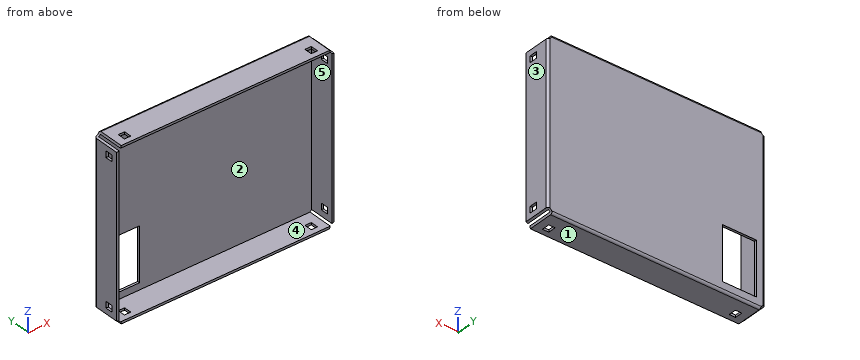
Autodesk Inventor part; units mm, degrees
ref_plane "YZ Plane" through (0, 0, 0) normal (1, 0, 0) x (0, 1, 0)
ref_plane "XZ Plane" through (0, 0, 0) normal (0, 1, 0) x (-1, 0, 0)
ref_plane "XY Plane" through (0, 0, 0) normal (0, 0, 1) x (1, 0, 0)
sketch "Sketch3" plane through (0, 0, 0) normal (0, 1, 0) x (-1, 0, 0)
  line L0 (23, 18.5) -> (-23, 18.5)
  line L1 (-24, 17.5) -> (-24, -17.5)
  line L2 (-23, -18.5) -> (23, -18.5)
  line L3 (24, -17.5) -> (24, 17.5)
  line L4 (24, 18.5) -> (-24, -18.5) construction
  circle A0 centre (24, 18.5) radius 1
  circle A1 centre (24, -18.5) radius 1
  circle A2 centre (-24, -18.5) radius 1
  circle A3 centre (-24, 18.5) radius 1
  point P0 (0, 0)
  dimension "d21" = 2
  dimension "d22" = 2
  dimension "d23" = 2
  dimension "d24" = 2
extrude "Extrusion3" add sketch "Sketch3" along normal blind 0.5 contours A0 L3 A1 L2 A2 L1 A3 L0
sketch "Sketch6" plane through (0, 0, 0) normal (0, -1, 0) x (1, 0, 0)
  line L0 (-23, 18.5) -> (23, 18.5)
  line L1 (-23, 18.5) -> (23, 18.5)
  line L2 (24, 17.5) -> (24, -17.5)
  line L3 (24, 17.5) -> (24, -17.5)
  line L4 (-24, -17.5) -> (-24, 17.5)
  line L5 (-24, -17.5) -> (-24, 17.5)
  circle A0 centre (-24, 18.5) radius 1
  circle A1 centre (24, 18.5) radius 1
  circle A2 centre (24, -18.5) radius 1
  circle A3 centre (-24, -18.5) radius 1
  line L6 (23.5, -17.634) -> (23.5, 17.634)
  line L7 (-23.134, 18) -> (23.134, 18)
  line L8 (-23.5, -17.634) -> (-23.5, 17.634)
  line L9 (23, -18.5) -> (-23, -18.5)
  line L10 (-23, -18.5) -> (23, -18.5)
  line L11 (23.134, -18) -> (-23.134, -18)
  point P0 (0, 0)
  dimension "d45" = 0.5
  dimension "d46" = 0.5
  dimension "d48" = 2
  dimension "d49" = 0.5
extrude "Extrusion5" add sketch "Sketch6" along normal blind 5.5 contours L0 A1 L7 A0 | A0 L8 A3 L4 | L2 A2 L6 A1 | A3 L11 A2 L9
sketch "Sketch7" plane through (-23, 0.5, 18.5) normal (0, 0, 1) x (1, 0, 0)
  line L0 (42.9, -3.1) -> (44.3, -3.1)
  line L1 (44.3, -3.1) -> (44.3, -4.8)
  line L2 (44.3, -4.8) -> (42.9, -4.8)
  line L3 (42.9, -4.8) -> (42.9, -3.1)
  line L4 (0, 0) -> (46, 0)
  line L5 (46, -6) -> (46, 0)
  line L6 (1.7, -3.1) -> (3.1, -3.1)
  line L7 (3.1, -3.1) -> (3.1, -4.8)
  line L8 (3.1, -4.8) -> (1.7, -4.8)
  line L9 (1.7, -4.8) -> (1.7, -3.1)
  line L10 (0, 0) -> (0, -6)
  point P0 (23, -0.5)
  dimension "d52" = 1.4
  dimension "d53" = 1.7
  dimension "d54" = 3.1
  dimension "d55" = 1.7
  dimension "d56" = 1.4
  dimension "d57" = 1.7
  dimension "d58" = 3.1
  dimension "d59" = 1.7
extrude "Extrusion6" cut sketch "Sketch7" against normal up to surface (37 mm away)
sketch "Sketch8" plane through (24, 0.5, 17.5) normal (1, 0, 0) x (0, 0, -1)
  line L0 (32.4, -3.1) -> (33.8, -3.1)
  line L1 (33.8, -3.1) -> (33.8, -4.8)
  line L2 (33.8, -4.8) -> (32.4, -4.8)
  line L3 (32.4, -4.8) -> (32.4, -3.1)
  line L4 (0, 0) -> (35, 0)
  line L5 (35, -6) -> (35, 0)
  line L6 (1.2, -3.1) -> (2.6, -3.1)
  line L7 (2.6, -3.1) -> (2.6, -4.8)
  line L8 (2.6, -4.8) -> (1.2, -4.8)
  line L9 (1.2, -4.8) -> (1.2, -3.1)
  line L10 (0, -6) -> (0, 0)
  point P0 (17.5, -0.5)
  dimension "d62" = 1.4
  dimension "d63" = 1.7
  dimension "d64" = 3.1
  dimension "d65" = 1.2
  dimension "d66" = 1.4
  dimension "d67" = 1.7
  dimension "d68" = 3.1
  dimension "d69" = 1.2
extrude "Extrusion7" cut sketch "Sketch8" against normal up to surface (48 mm away)
sketch "Sketch9" plane through (0, 0.5, 0) normal (0, 1, 0) x (1, 0, 0)
  line L0 (-22, 4.7) -> (-14.5, 4.7)
  line L1 (-14.5, 4.7) -> (-14.5, 16.5)
  line L2 (-14.5, 16.5) -> (-22, 16.5)
  line L3 (-22, 16.5) -> (-22, 4.7)
  line L4 (-24, 17.5) -> (-24, -17.5)
  line L5 (23, 18.5) -> (-23, 18.5)
  point P0 (0, 0)
  dimension "d74" = 7.5
  dimension "d75" = 11.8
  dimension "d76" = 2
  dimension "d77" = 2
extrude "Extrusion8" cut sketch "Sketch9" against normal up to surface (0.5 mm away)
fillet "Fillet1" radius 0.5 4 edges at (0, 0.5, -18.5) (24, 0.5, 0) (0, 0.5, 18.5) (-24, 0.5, 0)
properties part number "metal_cover_connector"
The listing builds one solid part. Answer for the finished solid, in the listing's coordinates (mm). Face numbers are marked on the shaded views. A direction names the side the tool comes from. Give positions to 0.01 mm unless a question says otherwise; leave off trailing zeros. Write each loop counter-clockwise with the first axis right and the second up, starting at its lowest first coordinate (ties: lowest second). Pieces come first, ordered by that corner, then holes.
Item 1: Section B-B, the plane z = -6 is taken. Write down the section's boundary in (x, y).
Item 2: Determine the mould class of the marked faces 3, 4 and 5 for opening direction X: released by +X, released by -X, zero draft, split by the parting line, or undercut.
Item 3: Which of the six approach directions +Z, -Z, +X, -X, +Y, -Y give full straight-line access (tool end or side, diameter ignored) to the marked faces 1 and 2?
Item 4: Section A-A, the plane x = -19 is taken. Write down the section's boundary in (y, z).
Item 5: Find the intervals of material crossed by line 1 along X through (y, z) = (-2.25, 8.5); line 2 along Z through (x, y) = (-1.5, -1.75); line 3 along Y through (x, z) = (11.5, 3), in increasing order.
Item 6: Section D-D, the plane x = 12.5 is taken. Write down the section's boundary in (y, z), plus the area to 3 significant figures.
Item 7: Flat-ended cylindrical pins translate along their axes: P1, Ø0.6, axis at y = -3.5, z = 18, coming from the -X side; P2, Ø3, axis at x = -15.5, z = 3.5, coming from the -Y side. Find the tip coordinate at first contact, or state that the pin passes through.
Item 8: Section C-C, the plane y = -1.25 is taken. Write down the section's boundary in (x, z), plus the area to 3 significant figures.
Completed:
1. outline: (-24, -5.5) - (-23.5, -5.5) - (-23.5, 0) - (-22, 0) - (-22, 0.5) - (-23.5, 0.5) arc R0.5 ccw to (-24, 0) - close; (-14.5, 0) - (23.5, 0) - (23.5, -5.5) - (24, -5.5) - (24, 0) arc R0.5 ccw to (23.5, 0.5) - (-14.5, 0.5) - close
2. face 3: released by +X
2. face 4: zero draft
2. face 5: undercut
3. face 1: -Z, +X, -X, +Y, -Y
3. face 2: -Y
4. outline: (-5.5, -18.5) - (0, -18.5) arc R0.5 ccw to (0.5, -18) - (0.5, -16.5) - (0, -16.5) - (0, -18) - (-5.5, -18) - close; (-5.5, 18) - (0, 18) - (0, -4.7) - (0.5, -4.7) - (0.5, 18) arc R0.5 ccw to (0, 18.5) - (-5.5, 18.5) - close
5. line 1: x = -24 to -23.5, 23.5 to 24
5. line 2: z = -18.5 to -18, 18 to 18.5
5. line 3: y = 0 to 0.5
6. outline: (-5.5, -18.5) - (0, -18.5) arc R0.5 ccw to (0.5, -18) - (0.5, 18) arc R0.5 ccw to (0, 18.5) - (-5.5, 18.5) - (-5.5, 18) - (0, 18) - (0, -18) - (-5.5, -18) - close
6. area: 23.9 mm2
7. P1: stops at x = -23.13
7. P2: stops at y = 0
8. outline: (-24, -17.5) arc R1 cw to (-23.5, -17.63) - (-23.5, 17.63) arc R1 cw to (-24, 17.5) - close; (-23.13, -18) arc R1 cw to (-23, -18.5) - (23, -18.5) arc R1 cw to (23.13, -18) - close; (-23.13, 18) - (23.13, 18) arc R1 cw to (23, 18.5) - (-23, 18.5) arc R1 cw to start; (23.5, -17.63) arc R1 cw to (24, -17.5) - (24, 17.5) arc R1 cw to (23.5, 17.63) - close
8. area: 81.2 mm2
